```python
from build123d import *

# Parameters (mm, degrees)
BOSS_EXTRUDE1_DEPTH     = 3.15
SKETCH2_R               = 1.75
BOSS_EXTRUDE2_DEPTH     = 1.15
FILLET1_R               = 0.2
SKETCH3_R               = 0.45
BOSS_EXTRUDE3_DEPTH     = 0.3
SKETCH4_W               = 0.7
SKETCH4_H               = 0.3
MIRROR2_COPY_1_SKETCH_W = 0.7
MIRROR2_COPY_1_SKETCH_H = 0.3
FILLET2_R               = 0.1


with BuildPart() as part:
    # Sketch1 → Boss-Extrude1 (new body)
    with BuildSketch(Plane(origin=(0, 0, 0), x_dir=(1, 0, 0), z_dir=(0, 1, 0))):
        with BuildLine():
            Line((-2.7, 3), (2.7, 3))
            ThreePointArc((2.7, 3), (2.912132034, 2.912132034), (3, 2.7))
            Line((3, 2.7), (3, -2.7))
            ThreePointArc((3, -2.7), (2.912132034, -2.912132034), (2.7, -3))
            Line((2.7, -3), (-2.7, -3))
            ThreePointArc((-2.7, -3), (-2.912132034, -2.912132034), (-3, -2.7))
            Line((-3, -2.7), (-3, 2.7))
            ThreePointArc((-3, 2.7), (-2.912132034, 2.912132034), (-2.7, 3))
        make_face()
    extrude(amount=BOSS_EXTRUDE1_DEPTH)

    # Sketch2 → Boss-Extrude2 (add)
    with BuildSketch(Plane(origin=(0, 3.15, 0), x_dir=(1, 0, 0), z_dir=(0, 1, 0))):
        with Locations(Location((0, 0, 0), (0, 0, 270))):
            Circle(SKETCH2_R)
    extrude(amount=BOSS_EXTRUDE2_DEPTH)

    # Fillet1
    fillet1_edges = [part.edges().sort_by_distance(p)[0] for p in [
        (0, 4.3, -1.75),
    ]]
    fillet(fillet1_edges, radius=FILLET1_R)

    # Sketch3 → Boss-Extrude3 (add)
    with BuildSketch(Plane(origin=(0, 3.15, 0), x_dir=(1, 0, 0), z_dir=(0, 1, 0))):
        with Locations(Location((-2.25, 2.25, 0), (0, 0, 270))):
            Circle(SKETCH3_R)
        with Locations(Location((2.25, 2.25, 0), (0, 0, 270))):
            Circle(SKETCH3_R)
        with Locations(Location((2.25, -2.25, 0), (0, 0, 270))):
            Circle(SKETCH3_R)
        with Locations(Location((-2.25, -2.25, 0), (0, 0, 270))):
            Circle(SKETCH3_R)
    extrude(amount=BOSS_EXTRUDE3_DEPTH)

    # Sweep1: sweep along a path in Sketch5
    with BuildLine(Plane.XY.offset(2.7)) as sweep1_path:
        Line((3, 0.5), (3.118975032, 0.5))
        ThreePointArc((3.118975032, 0.5), (3.289187664, 0.470135789), (3.439067232, 0.38411064))
        Line((3.439067232, 0.38411064), (3.760932768, 0.11588936))
        ThreePointArc((3.760932768, 0.11588936), (3.910812336, 0.029864211), (4.081024968, 0))
        Line((4.081024968, 0), (4.2, 0))
    # Sketch4 → Sweep1 (sweep)
    with BuildSketch(Plane(origin=(3, 0, 0), x_dir=(0, 0, -1), z_dir=(1, 0, 0))):
        with Locations((-2.35, 0.65)):
            Rectangle(SKETCH4_W, SKETCH4_H)
    sweep1 = sweep(path=sweep1_path.line)

    # Mirror1: Sweep1 across plane
    add(sweep1.mirror(Plane.XY))

    # Mirror2: Sweep1 across plane
    add(sweep1.mirror(Plane(origin=(0, 0, 0), x_dir=(0, 0, 1), z_dir=(1, 0, 0))))

    # Mirror2 copy 1: sweep along a path in Mirror2 copy 1 path
    with BuildLine(Plane(origin=(0, 0, -2.7), x_dir=(-1, 0, 0), z_dir=(0, 0, -1))) as mirror2_copy_1_path:
        Line((3, 0.5), (3.118975032, 0.5))
        ThreePointArc((3.118975032, 0.5), (3.289187664, 0.470135789), (3.439067232, 0.38411064))
        Line((3.439067232, 0.38411064), (3.760932768, 0.11588936))
        ThreePointArc((3.760932768, 0.11588936), (3.910812336, 0.029864211), (4.081024968, 0))
        Line((4.081024968, 0), (4.2, 0))
    # Mirror2 copy 1 sketch → Mirror2 copy 1 (sweep)
    with BuildSketch(Plane.ZY.offset(3)):
        with Locations((-2.35, 0.65)):
            Rectangle(MIRROR2_COPY_1_SKETCH_W, MIRROR2_COPY_1_SKETCH_H)
    sweep(path=mirror2_copy_1_path.line)

    # Fillet2
    fillet2_edges = [part.edges().sort_by_distance(p)[0] for p in [
        (-2.25, 3.45, -2.7),
        (2.25, 3.45, -2.7),
        (2.25, 3.45, 1.8),
        (-2.25, 3.45, 1.8),
    ]]
    fillet(fillet2_edges, radius=FILLET2_R)


solid = part.part
```
Here's how the part is built. I have some questions about the finished solid (model axes, mm). A direction names the side the tool comes from. Round coordinates to 2 decimals unless told otherwise and drop trailing zeros. Order: outer loops, then holes, each group sorted by start corner. A loop starts at its lowest first (then second) coordinate and runs counter-clockwise, first axis right, second up. Notation, with made-up numbers: M -1,66 L 54,66 A23 ccw 54,91 Z; hole C 66.5,33.5 d10. An arc over 180 degrees is marked long. Answer as CSV lines item,"result".
Item 1: For pin 1 (0.8 mm diameter, centred on x = 2, z = 2, fed in from +Y); pin 2 (0.6 mm diameter, centred on x = 3.5, y = 0.5, fed in from +Z); pin 3 (1.5 mm diameter, centred on y = 3.5, z = 1, fed in from -X), each with a flat end and sliding along its axis, tell me the tip position at first contact or that it passes through.
From the geometry:
pin 1,"y = 3.45"
pin 2,"z = 2.7"
pin 3,"x = -3"
Item 2: Which directions (+Z, -Z, +X, -X, +Y, -Y) give clear straight access to the entire face, cutting with the end or side of a thin tool? Please do faces 4 (the flat face through (0, 2, 3)), 5 (the cylindrical face through (-1.71, 3.62, -0.38)).
From the geometry:
face 4,"+Z, +X, -X, +Y, -Y"
face 5,"+Y"
Item 3: Imagine slicing it at D-D on x = 0. List the corners of the cut face in (y, z) for me.
From the geometry:
outline,"M 0,-3 L 3.15,-3 L 3.15,-1.75 L 4.1,-1.75 A0.2 ccw 4.3,-1.55 L 4.3,1.55 A0.2 ccw 4.1,1.75 L 3.15,1.75 L 3.15,3 L 0,3 Z"
Item 4: Please list where these lines run through material, in increasing order: L1, parallel to X at y = 2.85, z = -2; L2, parallel to Y at x = 2, z = -1.8; L3, parallel to Y at x = 0.25, z = -1.55. Write a range as [from, to].
From the geometry:
L1,"[-3, 3]"
L2,"[0, 3.15]"
L3,"[0, 4.3]"
Item 5: We'd pull the mould along Z, two halves only. Please class faces 1 (the flat face through (0, 2, -3)), 2 (the flat face through (0, 0, 0)), 3 (the flat face through (1.4, 3.15, -1.4)): +Z half, -Z half, draft (parallel to the pull), parting line (faces both ways), or undercut.
From the geometry:
face 1,"-Z half"
face 2,"draft"
face 3,"undercut"
Item 6: Imagine slicing it at C-C on y = 2. List the corners of the cut face in (x, z) for me.
From the geometry:
outline,"M -3,-2.7 A0.3 ccw -2.7,-3 L 2.7,-3 A0.3 ccw 3,-2.7 L 3,2.7 A0.3 ccw 2.7,3 L -2.7,3 A0.3 ccw -3,2.7 Z"
Item 7: Imagine slicing it at B-B on z = 0. List the corners of the cut face in (x, y) for me, and give its area (3 significant figures).
From the geometry:
outline,"M -3,0 L 3,0 L 3,3.15 L 1.75,3.15 L 1.75,4.1 A0.2 ccw 1.55,4.3 L -1.55,4.3 A0.2 ccw -1.75,4.1 L -1.75,3.15 L -3,3.15 Z"
area,"22.9 mm2"
Item 8: Imagine slicing it at A-A on x = -2.25. List the corners of the cut face in (y, z) for me.
From the geometry:
outline,"M 0,-3 L 3.15,-3 L 3.15,-2.7 L 3.35,-2.7 A0.1 ccw 3.45,-2.6 L 3.45,-1.9 A0.1 ccw 3.35,-1.8 L 3.15,-1.8 L 3.15,1.8 L 3.35,1.8 A0.1 ccw 3.45,1.9 L 3.45,2.6 A0.1 ccw 3.35,2.7 L 3.15,2.7 L 3.15,3 L 0,3 Z"
